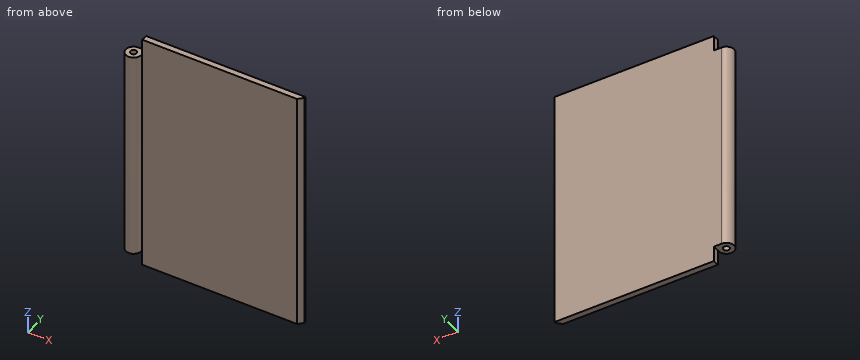
```python
from build123d import *

# Parameters (mm, degrees)
SKETCH1_R           = 2
BOSS_EXTRUDE1_DEPTH = 136
SKETCH2_W           = 104
SKETCH2_H           = 4
BOSS_EXTRUDE2_DEPTH = 10
SKETCH3_W           = 104
SKETCH3_H           = 4
BOSS_EXTRUDE3_DEPTH = 10
CUT_EXTRUDE2_DEPTH  = 191.373317458


with BuildPart() as part:
    # Sketch1 → Boss-Extrude1 (new body)
    with BuildSketch(Plane.XY):
        with BuildLine():
            Line((0, 5), (109, 5))
            Line((109, 5), (109, 1))
            Line((109, 1), (4.898979486, 1))
            ThreePointArc((4.898979486, 1), (-3.16227766, -3.872983346), (0, 5))
        make_face()
        Circle(SKETCH1_R, mode=Mode.SUBTRACT)
    extrude(amount=BOSS_EXTRUDE1_DEPTH)

    # Sketch2 → Boss-Extrude2 (add)
    with BuildSketch(Plane.XY.offset(136)):
        with Locations((57, 3)):
            Rectangle(SKETCH2_W, SKETCH2_H)
    extrude(amount=BOSS_EXTRUDE2_DEPTH)

    # Sketch3 → Boss-Extrude3 (add)
    with BuildSketch(Plane(origin=(0, 0, 0), x_dir=(-1, 0, 0), z_dir=(0, 0, -1))):
        with Locations((-57, 3)):
            Rectangle(SKETCH3_W, SKETCH3_H)
    extrude(amount=BOSS_EXTRUDE3_DEPTH)

    # Sketch5 → Cut-Extrude2 (cut, through all)
    with BuildSketch(Plane.XY.offset(146)):
        Polygon((106, 1), (109, 4), (109, 1), align=None)
    extrude(amount=-CUT_EXTRUDE2_DEPTH, mode=Mode.SUBTRACT)


solid = part.part
```
Read the model definition and answer for the solid it produces. Units are mm, in the model's axes. Round coordinates to 2 decimals unless told otherwise and drop trailing zeros. Loops run counter-clockwise (first coordinate to the right, second up) from the corner with the lowest first, then second, coordinate; pieces in that order, holes last. Notation, with made-up numbers: (-12, -26) -> (8, -26) arc R16 ccw to (8, -21) -> close; hole circle Ø11 at (14.5, 66.25). An arc over 180 degrees is marked (long way). One line per item, written item: value.
1) A cutting plane is placed at A-A (z = 67.5). Determine the outline of the cut face in (x, y), and give its area (3 significant figures).
Answer list:
outline: (0, 5) arc R5 ccw (long way) to (4.9, 1) -> (106, 1) -> (109, 4) -> (109, 5) -> close; hole circle Ø4 at (0, 0)
area: 483 mm²
2) Consider L1, parallel to Y at x = 22, z = 55.5; L2, parallel to X at y = 4, z = 136.5; L3, parallel to X at y = 0.25, z = 48. Determine where each line is inside the solid, lowest interval first. Write a range as [from, to].
Answer list:
L1: y = [1, 5]
L2: x = [5, 109]
L3: x = [-4.99, -1.98], [1.98, 4.99]
3) A cutting plane is placed at B-B (x = 77.5). Determine the outline of the cut face in (y, z).
Answer list:
outline: (1, -10) -> (5, -10) -> (5, 146) -> (1, 146) -> close
4) Flat-ended cylindrical pins translate along their axes: P1, Ø2, axis at x = 24, y = -1, coming from the +Z side; P2, Ø1.2, axis at y = 2, z = 139.5, coming from the -X side; P3, Ø2, axis at x = 29.5, z = 59.5, coming from the -Y side. Find the tip coordinate at first contact, or state that the pin passes through.
Answer list:
P1: passes through
P2: stops at x = 5
P3: stops at y = 1
